The listing builds one solid part. Answer for the finished solid, in the listing's coordinates (mm). Face numbers are marked on the shaded views. A direction names the side the tool comes from. Round coordinates to 2 decimals unless told otherwise and drop trailing zeros. Write each loop counter-clockwise with the first axis right and the second up, starting at its lowest first coordinate (ties: lowest second). Pieces come first, ordered by that corner, then holes. Notation, with made-up numbers: (-25, -27) - (-3, -27) arc R31 ccw to (-3, 1) - close; hole circle Ø3 at (-27, -15). An arc over 180 degrees is marked (long way). Answer in a Markdown table with one row per item.
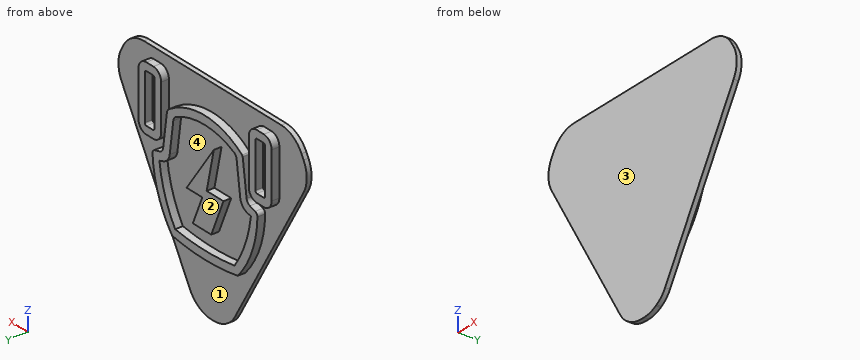
from build123d import *

# Parameters (mm, degrees)
SALIENTE_EXTRUIR1_DEPTH   = 4
SALIENTE_EXTRUIR1_2_DEPTH = 4
SALIENTE_EXTRUIR1_3_DEPTH = 4
SALIENTE_EXTRUIR1_4_DEPTH = 4
SALIENTE_EXTRUIR4_DEPTH   = 2.5


with BuildPart() as part:
    # Croquis1 → Saliente-Extruir1 (new body)
    with BuildSketch(Plane(origin=(0, 0, 0), x_dir=(1, 0, 0), z_dir=(0, 1, 0))):
        with BuildLine():
            ThreePointArc((24.735317162, -10.364213377), (24.248592978, -11.720458271), (23.256713943, -12.765674337))
            ThreePointArc((23.256713943, -12.765674337), (-0.301443486, -19.95898411), (-23.6872801, -12.223796151))
            ThreePointArc((-23.6872801, -12.223796151), (-23.957956222, -11.928413602), (-24.090963646, -11.550491071))
            Line((-24.090963646, -11.550491071), (-26.593504351, 6.639690423))
            ThreePointArc((-26.593504351, 6.639690423), (-27.283319128, 8.17801652), (-28.693873074, 9.101395733))
            Line((-28.693873074, 9.101395733), (-32.150547194, 10.150996156))
            ThreePointArc((-32.150547194, 10.150996156), (-33.187437723, 10.889076251), (-33.569084317, 12.103263251))
            ThreePointArc((-33.569084317, 12.103263251), (-30.118383627, 29.630783624), (-20.863266874, 44.910316325))
            ThreePointArc((-20.863266874, 44.910316325), (0.239054347, 46.767665402), (21.341375569, 44.910316325))
            ThreePointArc((21.341375569, 44.910316325), (30.311360731, 29.654768569), (33.971770868, 12.340214899))
            ThreePointArc((33.971770868, 12.340214899), (33.591964571, 11.071163494), (32.502360075, 10.317833331))
            Line((32.502360075, 10.317833331), (29.306873174, 9.442473887))
            ThreePointArc((29.306873174, 9.442473887), (27.844705893, 8.527958517), (27.127684399, 6.959471444))
            Line((27.127684399, 6.959471444), (24.735317162, -10.364213377))
        make_face()
        with BuildLine():
            Line((20.603314318, -8.570902391), (22.906419095, 8.106412307))
            ThreePointArc((22.906419095, 8.106412307), (24.243847943, 11.130514009), (26.980259101, 12.986843989))
            Line((26.980259101, 12.986843989), (29.51197218, 13.81713433))
            ThreePointArc((29.51197218, 13.81713433), (26.070313597, 28.043115781), (19.407293404, 41.074912432))
            ThreePointArc((19.407293404, 41.074912432), (0.273848763, 42.495848638), (-18.859595878, 41.074912432))
            ThreePointArc((-18.859595878, 41.074912432), (-25.76543723, 27.985894011), (-29.361445326, 13.630345475))
            Line((-29.361445326, 13.630345475), (-27.064825612, 13.093562644))
            ThreePointArc((-27.064825612, 13.093562644), (-23.995371379, 11.292144095), (-22.48638433, 8.068851342))
            Line((-22.48638433, 8.068851342), (-20.161283591, -8.830099253))
            ThreePointArc((-20.161283591, -8.830099253), (-19.632507369, -10.162063132), (-18.546205688, -11.096772031))
            ThreePointArc((-18.546205688, -11.096772031), (0.060689408, -15.579037847), (18.697865881, -11.224396063))
            ThreePointArc((18.697865881, -11.224396063), (19.979160972, -10.133592829), (20.603314318, -8.570902391))
        make_face(mode=Mode.SUBTRACT)
    extrude(amount=SALIENTE_EXTRUIR1_DEPTH)



with BuildPart() as body_2:
    # Croquis1 → Saliente-Extruir1 2 (new body)
    with BuildSketch(Plane(origin=(0, 0, 0), x_dir=(1, 0, 0), z_dir=(0, 1, 0))):
        Polygon((-11.705967947, 14.426136366), (-0.899048263, 14.426136366), (-5.508070268, -6.59896119), (12.002660496, 18.633842358), (1.904898556, 18.633842358), (8.015220238, 33.347588292), (-3.8482709, 33.347588292), align=None)
    extrude(amount=SALIENTE_EXTRUIR1_2_DEPTH)


with BuildPart() as body_3:
    # Croquis1 → Saliente-Extruir1 3 (new body)
    with BuildSketch(Plane(origin=(0, 0, 0), x_dir=(1, 0, 0), z_dir=(0, 1, 0))):
        with BuildLine():
            Line((-33.018215507, -27.970809887), (-37.703834023, -27.970809887))
            ThreePointArc((-37.703834023, -27.970809887), (-41.239367929, -26.506343793), (-42.703834023, -22.970809887))
            Line((-42.703834023, -22.970809887), (-42.703834023, 0.725352507))
            ThreePointArc((-42.703834023, 0.725352507), (-41.239367929, 4.260886413), (-37.703834023, 5.725352507))
            Line((-37.703834023, 5.725352507), (-33.018215507, 5.725352507))
            ThreePointArc((-33.018215507, 5.725352507), (-29.482681601, 4.260886413), (-28.018215507, 0.725352507))
            Line((-28.018215507, 0.725352507), (-28.018215507, -22.970809887))
            ThreePointArc((-28.018215507, -22.970809887), (-29.482681601, -26.506343793), (-33.018215507, -27.970809887))
        make_face()
        with BuildLine():
            ThreePointArc((-33.230214616, -23.921699906), (-32.523107835, -23.628806688), (-32.230214616, -22.921699906))
            Line((-32.230214616, -22.921699906), (-32.230214616, 0.414545051))
            ThreePointArc((-32.230214616, 0.414545051), (-32.523107835, 1.121651832), (-33.230214616, 1.414545051))
            Line((-33.230214616, 1.414545051), (-37.542643739, 1.414545051))
            ThreePointArc((-37.542643739, 1.414545051), (-38.24975052, 1.121651832), (-38.542643739, 0.414545051))
            Line((-38.542643739, 0.414545051), (-38.542643739, -22.921699906))
            ThreePointArc((-38.542643739, -22.921699906), (-38.24975052, -23.628806688), (-37.542643739, -23.921699906))
            Line((-37.542643739, -23.921699906), (-33.230214616, -23.921699906))
        make_face(mode=Mode.SUBTRACT)
    extrude(amount=SALIENTE_EXTRUIR1_3_DEPTH)


with BuildPart() as body_4:
    # Croquis1 → Saliente-Extruir1 4 (new body)
    with BuildSketch(Plane(origin=(0, 0, 0), x_dir=(1, 0, 0), z_dir=(0, 1, 0))):
        with BuildLine():
            Line((43.03056828, -22.990060864), (43.03056828, 0.457791938))
            ThreePointArc((43.03056828, 0.457791938), (41.566102186, 3.993325844), (38.03056828, 5.457791938))
            Line((38.03056828, 5.457791938), (33.431492806, 5.457791938))
            ThreePointArc((33.431492806, 5.457791938), (29.8959589, 3.993325844), (28.431492806, 0.457791938))
            Line((28.431492806, 0.457791938), (28.431492806, -22.990060864))
            ThreePointArc((28.431492806, -22.990060864), (29.8959589, -26.52559477), (33.431492806, -27.990060864))
            Line((33.431492806, -27.990060864), (38.03056828, -27.990060864))
            ThreePointArc((38.03056828, -27.990060864), (41.566102186, -26.52559477), (43.03056828, -22.990060864))
        make_face()
        with BuildLine():
            Line((32.681003043, -22.909445085), (32.681003043, 0.429273953))
            ThreePointArc((32.681003043, 0.429273953), (32.973896262, 1.136380734), (33.681003043, 1.429273953))
            Line((33.681003043, 1.429273953), (37.969534376, 1.429273953))
            ThreePointArc((37.969534376, 1.429273953), (38.676641157, 1.136380734), (38.969534376, 0.429273953))
            Line((38.969534376, 0.429273953), (38.969534376, -22.909445085))
            ThreePointArc((38.969534376, -22.909445085), (38.676641157, -23.616551866), (37.969534376, -23.909445085))
            Line((37.969534376, -23.909445085), (33.681003043, -23.909445085))
            ThreePointArc((33.681003043, -23.909445085), (32.973896262, -23.616551866), (32.681003043, -22.909445085))
        make_face(mode=Mode.SUBTRACT)
    extrude(amount=SALIENTE_EXTRUIR1_4_DEPTH)


with BuildPart() as part_1:
    add(part.part)

    add(body_2.part)  # Saliente-Extruir4 merges body 2

    add(body_3.part)  # Saliente-Extruir4 merges body 3

    add(body_4.part)  # Saliente-Extruir4 merges body 4
    # Croquis4 → Saliente-Extruir4 (add)
    with BuildSketch(Plane.XZ):
        with BuildLine():
            Line((-43.946678981, 33.550376808), (44.509741085, 33.550376808))
            ThreePointArc((44.509741085, 33.550376808), (51.998021732, 31.547516992), (57.486572192, 26.073797202))
            Line((57.486572192, 26.073797202), (58.879911857, 23.670484273))
            ThreePointArc((58.879911857, 23.670484273), (60.903025841, 16.187650298), (58.920434856, 8.693977802))
            Line((58.920434856, 8.693977802), (14.830934948, -68.31152391))
            ThreePointArc((14.830934948, -68.31152391), (12.450857587, -71.434275551), (9.341944939, -73.83240153))
            Line((9.341944939, -73.83240153), (8.830099524, -74.129408577))
            ThreePointArc((8.830099524, -74.129408577), (5.205365249, -75.63859627), (1.313165605, -76.155440525))
            Line((1.313165605, -76.155440525), (-0.526820951, -76.156842617))
            ThreePointArc((-0.526820951, -76.156842617), (-4.419803759, -75.645930765), (-8.046833861, -74.142269004))
            Line((-8.046833861, -74.142269004), (-8.559131327, -73.846042366))
            ThreePointArc((-8.559131327, -73.846042366), (-11.671695164, -71.452657228), (-14.056528907, -68.333536506))
            Line((-14.056528907, -68.333536506), (-58.32332823, 8.709094133))
            ThreePointArc((-58.32332823, 8.709094133), (-60.317329602, 16.205451495), (-58.299908193, 23.695540015))
            Line((-58.299908193, 23.695540015), (-56.929239256, 26.063906519))
            ThreePointArc((-56.929239256, 26.063906519), (-51.439911073, 31.544662969), (-43.946678981, 33.550376808))
        make_face()
    extrude(amount=SALIENTE_EXTRUIR4_DEPTH)


solid = part_1.part
(1) Section C-C (z = -22) is taken. Give the vertices of the cut face in (x, y).
Checked values:
| item | result |
|---|---|
| outline | (-40.68, -2.5) - (41.35, -2.5) - (41.35, 0) - (32.65, 0) - (32.65, 4) - (27.97, 4) - (27.97, 0) - (3.3, 0) - (3.3, 4) - (-8.56, 4) - (-8.56, 0) - (-27.71, 0) - (-27.71, 4) - (-32.41, 4) - (-32.41, 0) - (-40.68, 0) - close |
(2) Find the intervals of material crossed by line 1 (X direction, y = 1.5, z = -18.5); line 2 (X direction, y = 1.25, z = -28.5); line 3 (Z direction, x = 17.5, y = 1.5), in increasing order.
Checked values:
| item | result |
|---|---|
| line 1 | x = -33.04 to -28.55, -10.01 to 11.91, 28.77 to 33.33 |
| line 2 | x = -30.54 to -25.57, -5.86 to 6, 25.9 to 30.74 |
| line 3 | z = -45.53 to -41.35, 11.8 to 16.08 |
(3) For the marked faces 1 and 2, determine the directions among +Z, -Z, +X, -X, +Y, -Y from which every point of the face is accessible in a straight line to the end or side of a thin tool.
Checked values:
| item | result |
|---|---|
| face 1 | +Y |
| face 2 | +Z, -Z, +X, -X, +Y |
(4) Section A-A (y = -1.25) is taken. Give the vertices of the cut face in (x, z).
Checked values:
| item | result |
|---|---|
| outline | (-58.32, 8.71) - (-14.06, -68.33) arc R15 ccw to (-8.56, -73.85) - (-8.05, -74.14) arc R15 ccw to (-0.53, -76.16) - (1.31, -76.16) arc R15 ccw to (8.83, -74.13) - (9.34, -73.83) arc R15 ccw to (14.83, -68.31) - (58.92, 8.69) arc R15 ccw to (58.88, 23.67) - (57.49, 26.07) arc R15 ccw to (44.51, 33.55) - (-43.95, 33.55) arc R15 ccw to (-56.93, 26.06) - (-58.3, 23.7) arc R15 ccw to start |
(5) For a pull along Z with two mould halves and no side action, classify the marked faces 3 and 4 as pulls with the +Z half, pulls with the -Z half, needs draft (parallel to the pull), parting line crosses it, or undercut.
Checked values:
| item | result |
|---|---|
| face 3 | needs draft |
| face 4 | undercut |
(6) Flat-ended cylindrical pins translate along their axes: pin 1 (1.2 mm diameter, centred on x = -36, y = 3, fed in from -Z); pin 2 (1.2 mm diameter, centred on x = 35, y = 2, fed in from +Z); pin 3 (2 mm diameter, centred on y = 2, z = 11, fed in from +X). Find the tip coordinate at first contact, or state that the pin passes through.
Checked values:
| item | result |
|---|---|
| pin 1 | stops at z = -5.73 |
| pin 2 | stops at z = 27.99 |
| pin 3 | stops at x = 43.03 |
(7) Section D-D (z = -52) is taken. Give the vertices of the cut face in (x, y).
Checked values:
| item | result |
|---|---|
| outline | (-23.44, -2.5) - (24.17, -2.5) - (24.17, 0) - (-23.44, 0) - close |
(8) Section B-B (z = -35) is taken. Give the vertices of the cut face in (x, y) (3 decimals), and give its area (3 significant figures).
Checked values:
| item | result |
|---|---|
| outline | (-33.209, -2.5) - (33.903, -2.5) - (33.903, 0) - (27.903, 0) - (27.903, 4) - (22.997, 4) - (22.997, 0) - (-22.567, 0) - (-22.567, 4) - (-27.675, 4) - (-27.675, 0) - (-33.209, 0) - close |
| area | 208 mm2 |
